from build123d import *

# Parameters (mm, degrees)
SKETCH1_R                = 35
BOSS_EXTRUDE1_DEPTH      = 10
BOSS_EXTRUDE3_DEPTH      = 15
SKETCH3_R                = 25
CUT_EXTRUDE1_DEPTH       = 58
SKETCH4_R                = 35
BOSS_EXTRUDE5_DEPTH      = 10
SKETCH8_R                = 17.5
CUT_EXTRUDE4_DEPTH       = 201.5
SKETCH9_R                = 35
SKETCH9_R_2              = 25
BOSS_EXTRUDE7_DEPTH      = 10
BOSS_EXTRUDE8_DEPTH      = 7.5
CUT_EXTRUDE5_DEPTH       = 7.5
CUT_EXTRUDE15_DEPTH      = 91
CUT_EXTRUDE16_DEPTH      = 91
SKETCH21_W               = 4.689110868
SKETCH21_H               = 15
CUT_EXTRUDE17_DEPTH      = 40
CUT_EXTRUDE17_DEPTH_BACK = 30


with BuildPart() as part:
    # Sketch1 → Boss-Extrude1 (new body)
    with BuildSketch(Plane.XY):
        Circle(SKETCH1_R)
    extrude(amount=BOSS_EXTRUDE1_DEPTH)

    # Sketch2 → Boss-Extrude3 (add)
    with BuildSketch(Plane.XY.offset(10)):
        with BuildLine():
            Line((-30.310889132, 17.5), (-30.310889132, -17.5))
            ThreePointArc((-30.310889132, -17.5), (35, 0), (-30.310889132, 17.5))
        make_face()
    extrude(amount=BOSS_EXTRUDE3_DEPTH)

    # Sketch3 → Cut-Extrude1 (cut)
    with BuildSketch(Plane.XY.offset(25)):
        Circle(SKETCH3_R)
    extrude(amount=-CUT_EXTRUDE1_DEPTH, mode=Mode.SUBTRACT)

    # Sketch4 → Boss-Extrude5 (add)
    with BuildSketch(Plane.XY.offset(25)):
        Circle(SKETCH4_R)
    extrude(amount=BOSS_EXTRUDE5_DEPTH)

    # Sketch8 → Cut-Extrude4 (cut)
    with BuildSketch(Plane.XY.offset(35)):
        Circle(SKETCH8_R)
    extrude(amount=-CUT_EXTRUDE4_DEPTH, mode=Mode.SUBTRACT)

    # Sketch9 → Boss-Extrude7 (add)
    with BuildSketch(Plane.XY.offset(35)):
        Circle(SKETCH9_R)
        Circle(SKETCH9_R_2, mode=Mode.SUBTRACT)
    extrude(amount=BOSS_EXTRUDE7_DEPTH)

    # Sketch10 → Boss-Extrude8 (add)
    with BuildSketch(Plane.XY.offset(45)):
        with BuildLine():
            Line((-31.836956522, 14.539883061), (-20.336956522, 14.539883061))
            ThreePointArc((-20.336956522, 14.539883061), (0, 25), (20.336956522, 14.539883061))
            Line((20.336956522, 14.539883061), (31.836956522, 14.539883061))
            ThreePointArc((31.836956522, 14.539883061), (0, 35), (-31.836956522, 14.539883061))
        make_face()
        with BuildLine():
            Line((-31.836956522, -14.539883061), (-20.336956522, -14.539883061))
            ThreePointArc((-20.336956522, -14.539883061), (0, -25), (20.336956522, -14.539883061))
            Line((20.336956522, -14.539883061), (31.836956522, -14.539883061))
            ThreePointArc((31.836956522, -14.539883061), (0, -35), (-31.836956522, -14.539883061))
        make_face()
    extrude(amount=BOSS_EXTRUDE8_DEPTH)

    # Sketch11 → Cut-Extrude5 (cut)
    with BuildSketch(Plane.XY.offset(52.5)):
        with BuildLine():
            Line((-12.990381057, -32.5), (12.990381057, -32.5))
            ThreePointArc((12.990381057, -32.5), (0, -35), (-12.990381057, -32.5))
        make_face()
        with BuildLine():
            Line((-12.990381057, 32.5), (12.990381057, 32.5))
            ThreePointArc((12.990381057, 32.5), (0, 35), (-12.990381057, 32.5))
        make_face()
    extrude(amount=-CUT_EXTRUDE5_DEPTH, mode=Mode.SUBTRACT)

    # Sketch19 → Cut-Extrude15 (cut)
    with BuildSketch(Plane.XY.offset(45)):
        with BuildLine():
            Line((-5, 34.641016151), (-5, 32.5))
            Line((-5, 32.5), (5, 32.5))
            Line((5, 32.5), (5, 34.641016151))
            ThreePointArc((5, 34.641016151), (0, 35), (-5, 34.641016151))
        make_face()
    extrude(amount=-CUT_EXTRUDE15_DEPTH, mode=Mode.SUBTRACT)

    # Sketch20 → Cut-Extrude16 (cut)
    with BuildSketch(Plane.XY.offset(45)):
        with BuildLine():
            Line((-5, -34.641016151), (-5, -32.5))
            Line((-5, -32.5), (5, -32.5))
            Line((5, -32.5), (5, -34.641016151))
            ThreePointArc((5, -34.641016151), (0, -35), (-5, -34.641016151))
        make_face()
    extrude(amount=-CUT_EXTRUDE16_DEPTH, mode=Mode.SUBTRACT)

    # Sketch21 → Cut-Extrude17 (cut, two sides)
    with BuildSketch(Plane(origin=(0, 0, 0), x_dir=(1, 0, 0), z_dir=(0, 1, 0))) as cut_extrude17_sk:
        with Locations((32.655444566, -17.5)):
            Rectangle(SKETCH21_W, SKETCH21_H)
    extrude(amount=CUT_EXTRUDE17_DEPTH, mode=Mode.SUBTRACT)
    extrude(cut_extrude17_sk.sketch, amount=-CUT_EXTRUDE17_DEPTH_BACK, mode=Mode.SUBTRACT)


solid = part.part
CAD build for the part. Positions are in the model's coordinates, mm. A direction names the side the tool comes from. Round coordinates to 2 decimals unless told otherwise and drop trailing zeros. Write each loop counter-clockwise with the first axis right and the second up, starting at its lowest first coordinate (ties: lowest second). Pieces come first, ordered by that corner, then holes. Notation, with made-up numbers: M 59,-39.5 L 114,-39.5 A17 cw 114,-16.5 Z; hole C -27,19 d7. An arc over 180 degrees is marked long. Use a Markdown table: item, result. Add a question column.
1. Pull direction X, two halves, no side cores. Call faces 1 (the face through (-30.311, 0, 17)), 2 (the face through (5, 34, 23)), 3 (the face through (-29, 0, 45)): released by +X, released by -X, zero draft, split by the parting line, or undercut.
2. Slice it at C-C on x = 0. Give the cut face in (y, z), then the cut area to 4 significant figures.
3. Flat gauge pins, fed straight in: P1, Ø6, axis at x = 25.5, z = 47.5, coming from the -Y side; P2, Ø13, axis at x = -4, z = 31.5, coming from the +Y side; P3, Ø4, axis at y = -16, z = 42, coming from the +X side. Where does each tip first touch, or does it go through?
4. Slice it at B-B on z = 13. Give the cut face in (x, y).
5. Slice it at A-A on y = 0. Give the cut face in (x, z).
6. Slice it at D-D on z = 30.5. Give the cut face in (x, y).
7. 3-axis set-ups, long thin cutter, end or side, ignore diameter. For faces 4 (the face through (5, -34, 23)), 5 (the face through (26, -14.54, 49)), 6 (the face through (30.311, 0, 18)): which of +Z, -Z, +X, -X, +Y, -Y reach the whole face in a straight line?
8. Drill centre lines: probe 1 along Y at (x, z) = (0, 38.5); probe 2 along X at (y, z) = (9.5, 21.5); probe 3 along Y at (x, z) = (-12.5, 7). Where is each one in solid material? Low to high.
Reply:
| question | item | result |
|---|---|---|
| 1 | face 1 | released by -X |
| 1 | face 2 | undercut |
| 1 | face 3 | zero draft |
| 2 | outline | M -32.5,0 L -25,0 L -25,25 L -17.5,25 L -17.5,35 L -25,35 L -25,52.5 L -32.5,52.5 Z; M 17.5,25 L 25,25 L 25,0 L 32.5,0 L 32.5,52.5 L 25,52.5 L 25,35 L 17.5,35 Z |
| 2 | area | 937.5 mm^2 |
| 3 | P1 | stops at y = -26.81 |
| 3 | P2 | stops at y = 34.64 |
| 3 | P3 | stops at x = 32.08 |
| 4 | outline | M -30.31,-17.5 A35 ccw -5,-34.64 L -5,-32.5 L 5,-32.5 L 5,-34.64 A35 ccw 30.31,-17.5 L 30.31,17.5 A35 ccw 5,34.64 L 5,32.5 L -5,32.5 L -5,34.64 A35 ccw -30.31,17.5 Z; hole C 0,0 d50 |
| 5 | outline | M -35,0 L -25,0 L -25,25 L -17.5,25 L -17.5,35 L -25,35 L -25,45 L -35,45 L -35,25 L -30.31,25 L -30.31,10 L -35,10 Z; M 17.5,25 L 25,25 L 25,0 L 35,0 L 35,10 L 30.31,10 L 30.31,25 L 35,25 L 35,45 L 25,45 L 25,35 L 17.5,35 Z |
| 6 | outline | M -5,-34.64 L -5,-32.5 L 5,-32.5 L 5,-34.64 A35 ccw 5,34.64 L 5,32.5 L -5,32.5 L -5,34.64 A35 ccw Z; hole C 0,0 d35 |
| 7 | face 4 | +Z, -Z, -Y |
| 7 | face 5 | +Z, +X, -X |
| 7 | face 6 | +X, +Y, -Y |
| 8 | probe 1 | y = -32.5 to -25, 25 to 32.5 |
| 8 | probe 2 | x = -30.31 to -23.12, 23.12 to 30.31 |
| 8 | probe 3 | y = -32.69 to -21.65, 21.65 to 32.69 |
